CAD build for the part. Positions are in the model's coordinates, mm. Coordinates: 2 decimals unless noted, no trailing zeros. Write each loop counter-clockwise with the first axis right and the second up, starting at its lowest first coordinate (ties: lowest second). Pieces come first, ordered by that corner, then holes. Notation, with made-up numbers: M -13,-35 L -2,-35 A21 ccw -2,-28 Z; hole C 86,75 d10. An arc over 180 degrees is marked long. Put each result on its own line as item: value. Start each with the question number.
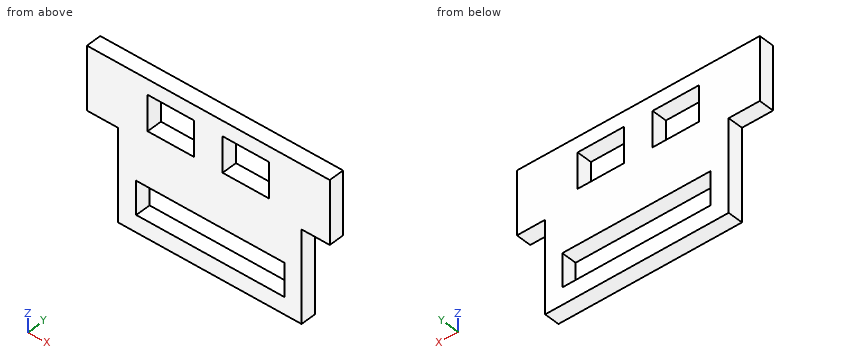
```python
from build123d import *

# Parameters (mm, degrees)
F0_W     = 101.399846375
F0_H     = 52.6096001267
F0_W_2   = 38.787077181
F0_H_2   = 29.5493621379
F1_DEPTH = 12.7
F3_W     = 153.2556563616
F3_H     = 76.6561478376
F3_W_2   = 123.7184926867
F3_H_2   = 27.7441889048
F4_DEPTH = 12.7


# Not quite as in the source:
# - the program builds the solid bodies; features that only make, move or delete a surface that nothing else refers to are left out


with BuildPart() as f1:
    # F0 (on Front) → F1 (new body)
    with BuildSketch(Plane.XZ):
        with Locations((-50.6999231875, 26.3048000634)):
            Rectangle(F0_W, F0_H)
        with Locations((-31.306384597, 25.2366727218)):
            Rectangle(F0_W_2, F0_H_2, mode=Mode.SUBTRACT)
    extrude(amount=F1_DEPTH)

    # F2: F1 across plane


with BuildPart() as f1_1:
    add(f1.part)
    add(f1.part.mirror(Plane.YZ))

    # F3 (on Front) → F4 (join)
    with BuildSketch(Plane.XZ):
        with Locations((1.2047663331, -38.3280739188)):
            Rectangle(F3_W, F3_H)
        with Locations((1.6441084445, -48.6036911607)):
            Rectangle(F3_W_2, F3_H_2, mode=Mode.SUBTRACT)
    extrude(amount=F4_DEPTH)


solid = f1_1.part
```
(1) Slice it at D-D, the plane z = -48. Write the cut outline in (x, y), then the cut area to 3 significant figures.
(2) Drop flat-ended pins along their axis: pin 1 (6.5 mm diameter, centred on y = -5.5, z = -28, fed in from -X); pin 2 (1 mm diameter, centred on y = -8.5, z = -19.5, fed in from +X). Give the stop position or say it passes through.
(3) Slice it at A-A, the plane z = 16. Write the cut outline in (x, y).
(4) Slice it at C-C, the plane y = -7.25. Write the cut outline in (x, z).
(5) Drill centre lines: line 1 (X direction, y = -9.75, z = 19); line 2 (Z direction, x = -42.5, y = -4.5); line 3 (X direction, y = -1.5, z = -54). Where is each one in solid material? Low to high. Write a range as [from, to].
(6) Slice it at B-B, the plane x = 48. Write the cut outline in (y, z), then the cut area to 3 significant figures.
Result set:
1. outline: M -75.42,-12.7 L -60.22,-12.7 L -60.22,0 L -75.42,0 Z; M 63.5,-12.7 L 77.83,-12.7 L 77.83,0 L 63.5,0 Z
1. area: 375 mm^2
2. pin 1: stops at x = -75.42
2. pin 2: stops at x = 77.83
3. outline: M -101.4,-12.7 L -50.7,-12.7 L -50.7,0 L -101.4,0 Z; M -11.91,-12.7 L 11.91,-12.7 L 11.91,0 L -11.91,0 Z; M 50.7,-12.7 L 101.4,-12.7 L 101.4,0 L 50.7,0 Z
4. outline: M -101.4,0 L -75.42,0 L -75.42,-76.66 L 77.83,-76.66 L 77.83,0 L 101.4,0 L 101.4,52.61 L -101.4,52.61 Z; hole M -60.22,-62.48 L 63.5,-62.48 L 63.5,-34.73 L -60.22,-34.73 Z; hole M -50.7,10.46 L -11.91,10.46 L -11.91,40.01 L -50.7,40.01 Z; hole M 11.91,10.46 L 50.7,10.46 L 50.7,40.01 L 11.91,40.01 Z
5. line 1: x = [-101.4, -50.7], [-11.91, 11.91], [50.7, 101.4]
5. line 2: z = [-76.66, -62.48], [-34.73, 10.46], [40.01, 52.61]
5. line 3: x = [-75.42, -60.22], [63.5, 77.83]
6. outline: M -12.7,-76.66 L 0,-76.66 L 0,-62.48 L -12.7,-62.48 Z; M -12.7,-34.73 L 0,-34.73 L 0,10.46 L -12.7,10.46 Z; M -12.7,40.01 L 0,40.01 L 0,52.61 L -12.7,52.61 Z
6. area: 914 mm^2
